Print and shaded views of the part. All mm, measured from the part's lowest x, y and z. A direction names the side the tool comes from. Coordinates: 2 decimals unless noted, no trailing zeros. One line per question, with ' | ' between items. Start each with the question number.
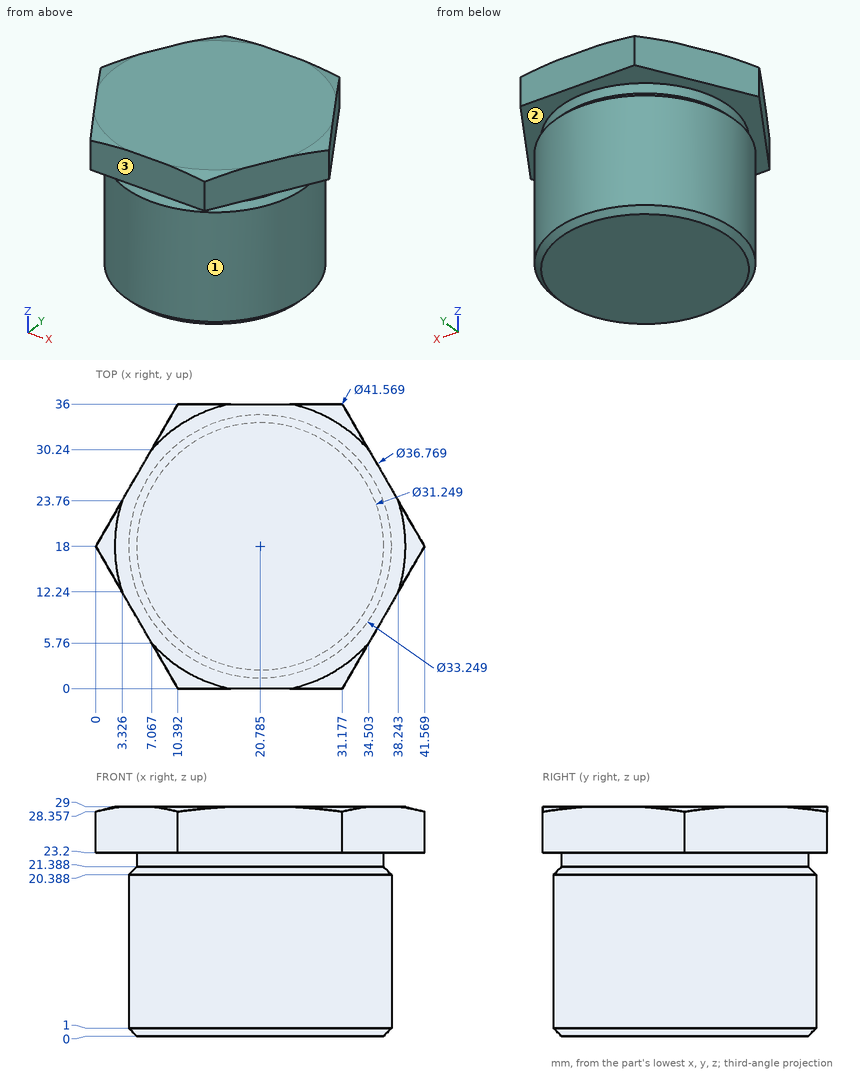
(1) Pin check, flat tips, straight feed: P1, Ø8, axis at x = 23.5, z = 10, coming from the -Y side (1 decimal); P2, Ø12, axis at x = 29.5, z = 5.5, coming from the -Y side; P3, Ø1, axis at y = 26, z = 15, coming from the +X side. Stop position of each tip, or through.
(2) Drill centre lines: line 1 (Y direction, x = 21, z = 13.75); line 2 (Z direction, x = 3, y = 18.5); line 3 (Z direction, x = 36, y = 22) (1 decimal). Where is each one in solid material? Low to high. Write a range as [from, to].
(3) 3-axis set-ups, long thin cutter, end or side, ignore diameter. For the marked faces 1, 2 and 3: which of +Z, -Z, +X, -X, +Y, -Y reach the whole face in a straight line?
Computed values:
1) P1: y = 1.4 | P2: y = 1.6 | P3: x = 35.62
2) line 1: [1.38, 34.62] | line 2: [23.2, 29] | line 3: [0.1, 21.3], [23.2, 29]
3) face 1: -Z | face 2: none | face 3: +Z, -Z, +X, -X, -Y
